The figure shows three views and two pictorial views of one solid part (mm, origin at its lowest corner). Answer the questions. A direction names the side the tool comes from. Give positions to 0.01 mm unless a question says otherwise; leave off trailing zeros. Write each loop counter-clockwise with the first axis right and the second up, starting at its lowest first coordinate (ties: lowest second). Pieces come first, ordered by that corner, then holes. Notation, with made-up numbers: (59.5, -35.5) - (99.5, -35.5) arc R22 cw to (99.5, -12.5) - close; hole circle Ø5 at (-15, -27.5). An arc over 180 degrees is marked (long way). Answer as CSV lines item,"result". Start each with the question number.
(1) Straight lines are drawn through the part: probe 1 along X at (y, z) = (6, 1.8); probe 2 along X at (y, z) = (8, 1.2); probe 3 along X at (y, z) = (1.5, 1.4). For each, find the intervals that lie inside material, in ascending order.
(2) Each of these flat-tipped pins is pushed along its axis until it touches: pin 1 Ø0.8 at (y, z) = (6.5, 1.5) entering from +X; pin 2 Ø0.8 at (y, z) = (6.5, 1.5) entering from -X; pin 3 Ø5.5 at (x, y) = (11.5, 4.5) entering from +Z; pin 4 Ø0.8 at (y, z) = (8, 0.5) entering from -X (3 decimals). Where does it stop, or does it pass through?
(3) Find section C-C (z = 0.3). Write down the section's boundary in (x, y).
(4) For a pull along X with two mould halves and no side action, classify the marked faces 3, 4, 5 and 6 as pulls with the +X half, pulls with the -X half, needs draft (parallel to the pull), parting line crosses it, or undercut.
(5) For the marked faces 1 and 2, determine the directions among +Z, -Z, +X, -X, +Y, -Y from which every point of the face is accessible in a straight line to the end or side of a thin tool.
(6) Find section B-B (z = 1.35). Write down the section's boundary in (x, y), then the cut area to 3 significant figures.
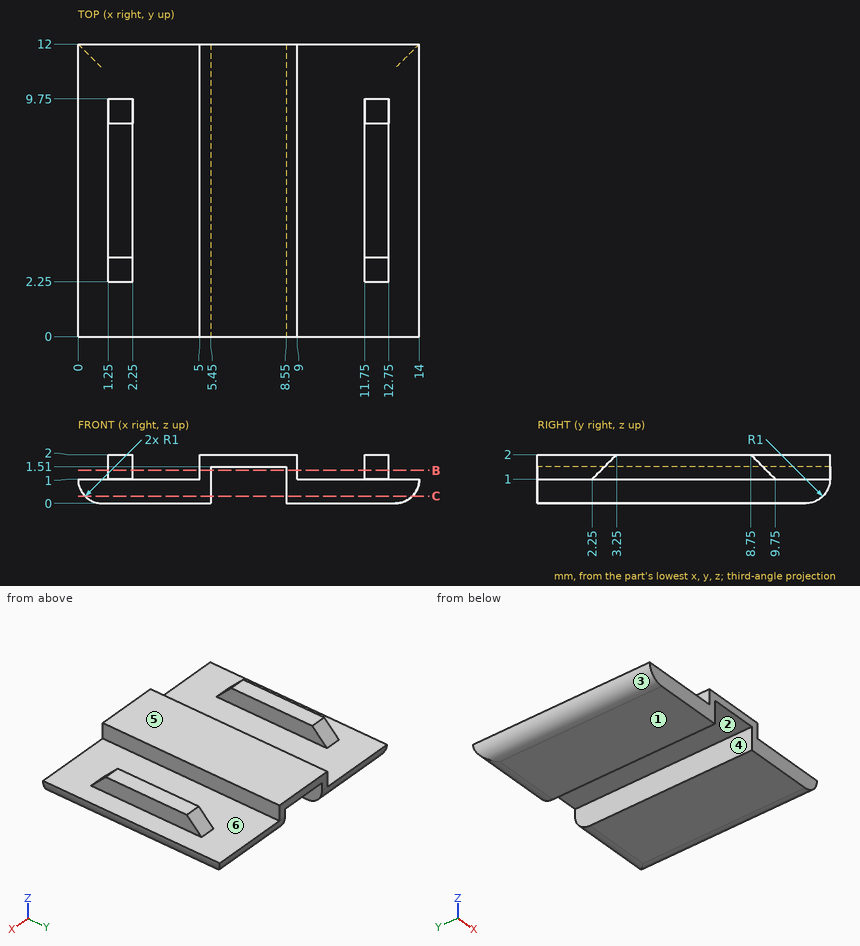
Result set:
1,probe 1,"1.25 to 2.25, 5 to 9, 11.75 to 12.75"
1,probe 2,"1.25 to 2.25, 5 to 5.45, 8.55 to 9, 11.75 to 12.75"
1,probe 3,"5 to 5.45, 8.55 to 9"
2,pin 1,"x = 12.75"
2,pin 2,"x = 1.25"
2,pin 3,"z = 2"
2,pin 4,"x = 0.005"
3,outline,"(0.29, 0) - (5.45, 0) - (5.45, 11.71) - (0.29, 11.71) - close; (8.55, 0) - (13.71, 0) - (13.71, 11.71) - (8.55, 11.71) - close"
4,face 3,"pulls with the -X half"
4,face 4,"undercut"
4,face 5,"needs draft"
4,face 6,"undercut"
5,face 1,"-Z, +X, -X, +Y, -Y"
5,face 2,"-Z, +Y, -Y"
6,outline,"(1.25, 2.6) - (2.25, 2.6) - (2.25, 9.4) - (1.25, 9.4) - close; (5, 0) - (5.45, 0) - (5.45, 12) - (5, 12) - close; (8.55, 0) - (9, 0) - (9, 12) - (8.55, 12) - close; (11.75, 2.6) - (12.75, 2.6) - (12.75, 9.4) - (11.75, 9.4) - close"
6,area,"24.4 mm^2"
